Source: three-view drawing plus pictorial views. Frame: mm from the lowest corner of the part. A direction names the side the tool comes from. Give positions to 0.01 mm unless a question says otherwise; leave off trailing zeros. Write each loop counter-clockwise with the first axis right and the second up, starting at its lowest first coordinate (ties: lowest second). Pieces come first, ordered by that corner, then holes. Notation, with made-up numbers: (30, 8.5) -> (76, 8.5) arc R20 cw to (76, 30.5) -> close; hole circle Ø2 at (66.5, -11.75). An arc over 180 degrees is marked (long way). Write item = value, one per line.
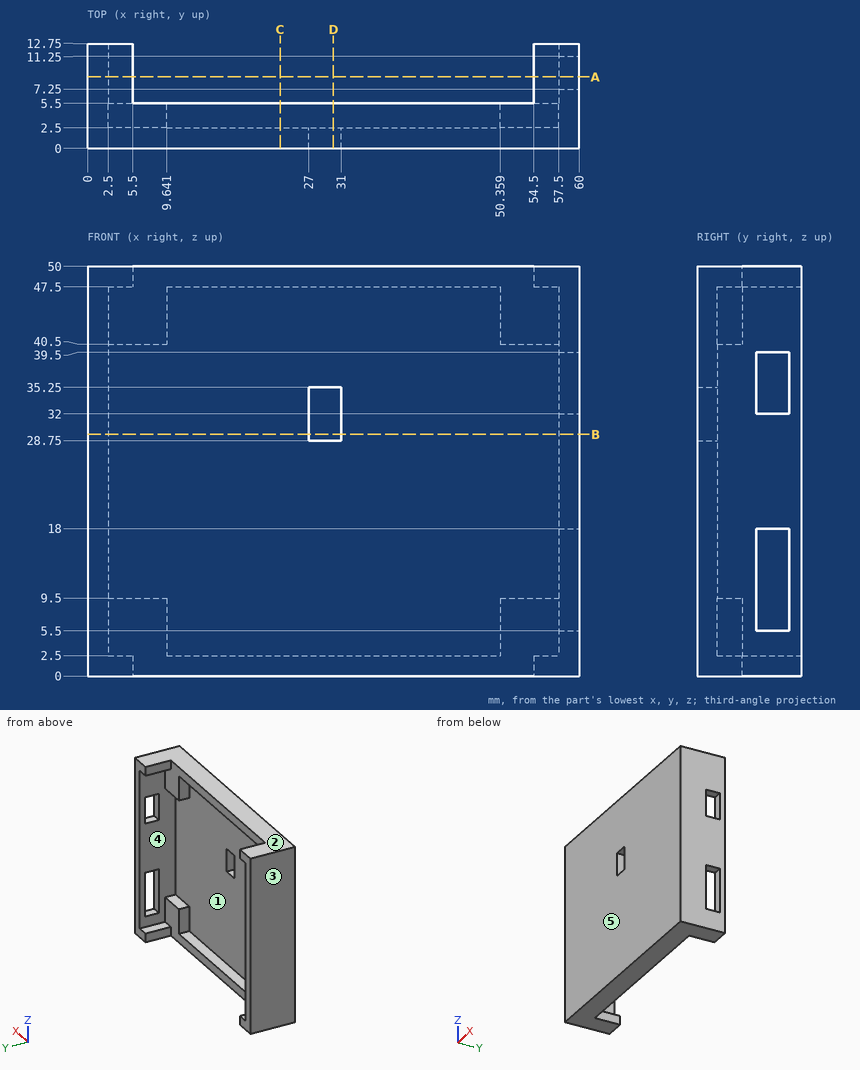
1) Access query for the marked faces 4 and 5. Directions: +Z, -Z, +X, -X, +Y, -Y. A direction counts if a zero-diameter tool reaches every point of the face in a straight line with its end or side. Return the directions, or none.
Computed:
face_4 = +Y
face_5 = +Z, -Z, +X, -X, -Y
2) Material intervals for L1, parallel to X at y = 12.25, z = 47; L2, parallel to X at y = 3.25, z = 3; L3, parallel to Z at x = 51.5, y = 3, sorted ascending.
Computed:
L1 = 0 to 2.5, 57.5 to 60
L2 = 0 to 9.64, 50.36 to 60
L3 = 0 to 9.5, 40.5 to 50
3) Cut plane A-A (y = 8.75). Return the cut outline in (x, z), then the cut area to 3 significant figures.
Computed:
outline = (0, 0) -> (5.5, 0) -> (5.5, 2.5) -> (2.5, 2.5) -> (2.5, 47.5) -> (5.5, 47.5) -> (5.5, 50) -> (0, 50) -> close; (54.5, 0) -> (60, 0) -> (60, 5.5) -> (57.5, 5.5) -> (57.5, 2.5) -> (54.5, 2.5) -> close; (54.5, 47.5) -> (57.5, 47.5) -> (57.5, 39.5) -> (60, 39.5) -> (60, 50) -> (54.5, 50) -> close; (57.5, 18) -> (60, 18) -> (60, 32) -> (57.5, 32) -> close
area = 230 mm²
4) Contact query for flat-ended pins moving along their axis: pin 1 (12 mm diameter, centred on x = 39.5, z = 31, fed in from +Y); pin 2 (2 mm diameter, centred on x = 36.5, y = 8, fed in from +Z). Output: stop coordinate, or through.
Computed:
pin_1 = 2.5
pin_2 = through
5) Draft query along Z for the marked faces 1, 2 and 3. Return one class per face: pulls with the +Z half, pulls with the -Z half, needs draft (parallel to the pull), parting line crosses it, or undercut.
Computed:
face_1 = undercut
face_2 = pulls with the +Z half
face_3 = needs draft
6) Cut plane B-B (z = 29.5). Return the cut outline in (x, y), then the cut area to 3 significant figures.
Computed:
outline = (0, 0) -> (27, 0) -> (27, 2.5) -> (2.5, 2.5) -> (2.5, 12.75) -> (0, 12.75) -> close; (31, 0) -> (60, 0) -> (60, 12.75) -> (57.5, 12.75) -> (57.5, 2.5) -> (31, 2.5) -> close
area = 191 mm²
7) Cut plane C-C (x = 23.5). Return the cut outline in (y, z).
Computed:
outline = (0, 0) -> (5.5, 0) -> (5.5, 2.5) -> (2.5, 2.5) -> (2.5, 47.5) -> (5.5, 47.5) -> (5.5, 50) -> (0, 50) -> close
8) Cut plane D-D (x = 30). Return the cut outline in (y, z).
Computed:
outline = (0, 0) -> (5.5, 0) -> (5.5, 2.5) -> (2.5, 2.5) -> (2.5, 28.75) -> (0, 28.75) -> close; (0, 35.25) -> (2.5, 35.25) -> (2.5, 47.5) -> (5.5, 47.5) -> (5.5, 50) -> (0, 50) -> close
